Answer from the drawing. Dimensions are ordinates in mm from the lowest x, y and z of the part. A direction names the side the tool comes from. Give positions to 0.01 mm unless a question says otherwise; leave off trailing zeros. Loops run counter-clockwise (first coordinate to the right, second up) from the corner with the lowest first, then second, coordinate; pieces in that order, holes last. Notation, with made-up numbers: (62.5, 34.25) -> (89.5, 34.25) arc R18 ccw to (89.5, 60.25) -> close; hole circle Ø1 at (-24, -20). An arc over 180 degrees is marked (long way). Return JSON: item names as keys, results as strings. Group by question number.
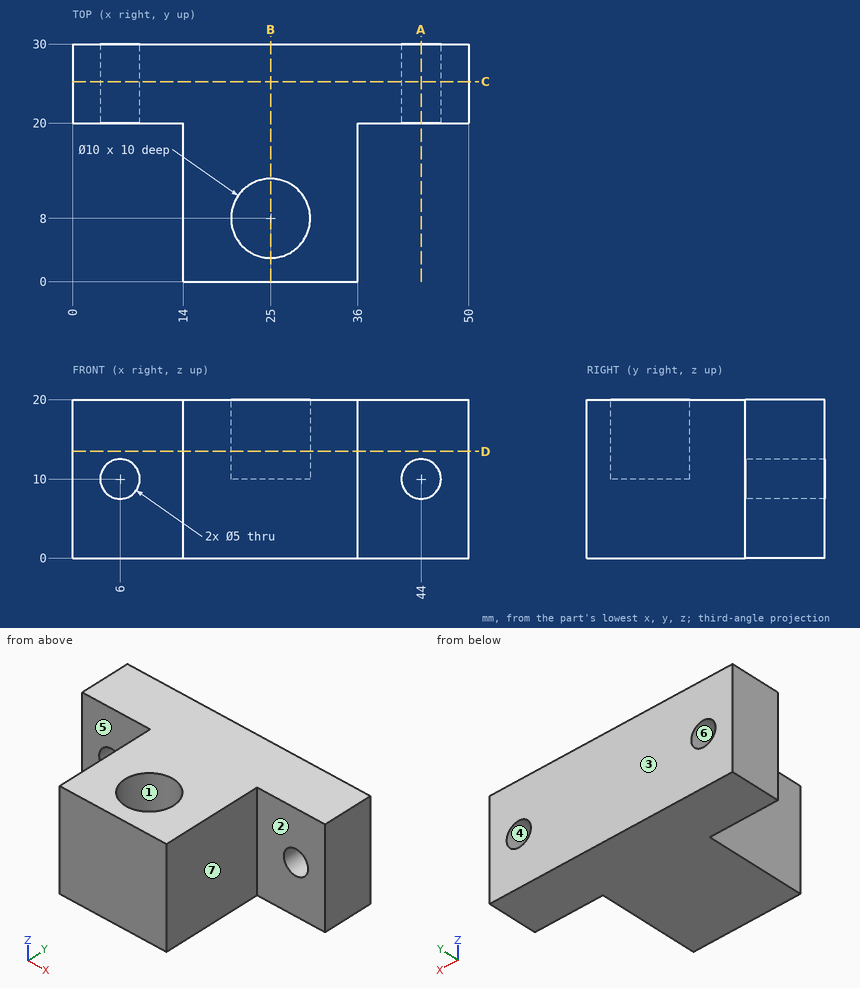
1. Section A-A on x = 44 is taken. Determine the outline of the cut face in (y, z).
2. Determine the mould class of the marked faces 1, 2, 3 and 4 for opening direction Y: pulls with the +Y half, pulls with the -Y half, needs draft (parallel to the pull), parting line crosses it, or undercut.
3. Flat-ended cylindrical pins translate along their axes: pin 1 Ø8 at (y, z) = (15, 7) entering from -X; pin 2 Ø6 at (y, z) = (10.5, 9.5) entering from +X; pin 3 Ø7 at (x, z) = (9, 14.5) entering from -Y. Find the tip coordinate at first contact, or state that the pin passes through.
4. Section C-C on y = 25.25 is taken. Determine the outline of the cut face in (x, z).
5. Section D-D on z = 13.5 is taken. Determine the outline of the cut face in (x, y), then the cut area to 3 significant figures.
6. Section B-B on x = 25 is taken. Determine the outline of the cut face in (y, z).
7. Straight lines are drawn through the part: line 1 (Z direction, x = 6, y = 27.5); line 2 (Y direction, x = 25, z = 16.25); line 3 (Y direction, x = 40, z = 18.75). For each, find the intervals that lie inside material, in ascending order. Write a range as from..to.
8. Which of the six approach directions +Z, -Z, +X, -X, +Y, -Y give full straight-line access (tool end or side, diameter ignored) to the marked faces 5, 6 and 7?
Completed:
{
 "1": {"outline": "(20, 0) -> (30, 0) -> (30, 7.5) -> (20, 7.5) -> close; (20, 12.5) -> (30, 12.5) -> (30, 20) -> (20, 20) -> close"},
 "2": {"face 1": "undercut", "face 2": "pulls with the -Y half", "face 3": "pulls with the +Y half", "face 4": "needs draft"},
 "3": {"pin 1": "stops at x = 14", "pin 2": "stops at x = 36", "pin 3": "stops at y = 20"},
 "4": {"outline": "(0, 0) -> (50, 0) -> (50, 20) -> (0, 20) -> close; hole circle Ø5 at (6, 10); hole circle Ø5 at (44, 10)"},
 "5": {"outline": "(0, 20) -> (14, 20) -> (14, 0) -> (36, 0) -> (36, 20) -> (50, 20) -> (50, 30) -> (0, 30) -> close; hole circle Ø10 at (25, 8)", "area": "861 mm²"},
 "6": {"outline": "(0, 0) -> (30, 0) -> (30, 20) -> (13, 20) -> (13, 10) -> (3, 10) -> (3, 20) -> (0, 20) -> close"},
 "7": {"line 1": "z = 0..7.5, 12.5..20", "line 2": "y = 0..3, 13..30", "line 3": "y = 20..30"},
 "8": {"face 5": "+Z, -Z, -X, -Y", "face 6": "+Y, -Y", "face 7": "+Z, -Z, +X, -Y"}
}
